Build history of the part. All positions in model axes, mm. Face numbers are marked on the shaded views. A direction names the side the tool comes from. Round coordinates to 2 decimals unless told otherwise and drop trailing zeros. Write each loop counter-clockwise with the first axis right and the second up, starting at its lowest first coordinate (ties: lowest second). Pieces come first, ordered by that corner, then holes. Notation, with made-up numbers: (85, 15.5) -> (125, 15.5) arc R7 ccw to (125, 28.5) -> close; hole circle Ø7 at (53.25, 53.25). An arc over 180 degrees is marked (long way). Return JSON: item names as keys, results as strings.
from build123d import *

# Parameters (mm, degrees)
F2_R     = 46.0375
F3_DEPTH = 19.05
F3_TAPER = 15
F0_R     = 41.275
F4_DEPTH = 25.4
F5_R     = 46.0375
F6_DEPTH = 1.5875


with BuildPart() as f3:
    # F2 (on offset) → F3 (new body)
    with BuildSketch(Plane.XY.offset(-41.275)):
        Circle(F2_R)
    extrude(amount=F3_DEPTH, taper=F3_TAPER)

    # F0 (on Top) → F4 (join)
    with BuildSketch(Plane.XY):
        Circle(F0_R)
    extrude(amount=-F4_DEPTH)

    # F5 (on face) → F6 (join)
    with BuildSketch(Plane(origin=(0, 0, -41.275), x_dir=(1, 0, 0), z_dir=(0, 0, -1))):
        Polygon((101.6, -101.6), (101.6, 0), (101.6, 101.6), (-101.6, 101.6), (-101.6, -101.6), align=None)
        Circle(F5_R, mode=Mode.SUBTRACT)
        Circle(F5_R)
    extrude(amount=F6_DEPTH)


solid = f3.part
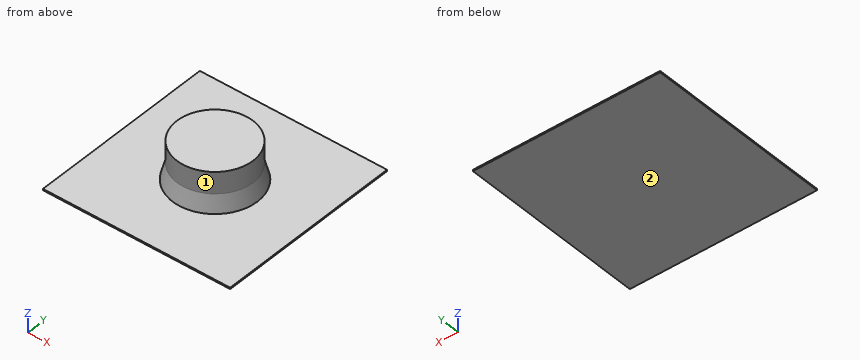
Q1. Saw through at D-D on y = 71. List the corners of the cut face in (x, z) (1 decimal).
Verdict:
{"outline": "(-101.6, -42.9) -> (101.6, -42.9) -> (101.6, -41.3) -> (-101.6, -41.3) -> close"}
Q2. Saw through at C-C on z = -5. List the corners of the cut face in (x, y) (3 decimals), then the cut area to 3 significant figures.
Verdict:
{"outline": "circle Ø82.55 at (0, 0)", "area": "5,350 mm²"}
Q3. Pin check, flat tips, straight feed: pin 1 Ø3 at (x, z) = (14.5, -23) entering from -Y; pin 2 Ø4 at (x, z) = (-20.5, -15) entering from -Y. Stop position of each tip, or through.
Verdict:
{"pin 1": "stops at y = -39.19", "pin 2": "stops at y = -36.9"}
Q4. 3-axis set-ups, long thin cutter, end or side, ignore diameter. For the marked faces 1 and 2: which of +Z, -Z, +X, -X, +Y, -Y reach the whole face in a straight line?
Verdict:
{"face 1": "+Z", "face 2": "-Z, +X, -X, +Y, -Y"}
Q5. Saw through at A-A on y = 0. List the corners of the cut face in (x, z) (1 decimal), then the cut area to 3 significant figures.
Verdict:
{"outline": "(-101.6, -42.9) -> (101.6, -42.9) -> (101.6, -41.3) -> (46, -41.3) -> (41.3, -23.5) -> (41.3, 0) -> (-41.3, 0) -> (-41.3, -23.5) -> (-46, -41.3) -> (-101.6, -41.3) -> close", "area": "3,810 mm²"}
Q6. Wall check: L1, parallel to Z at x = -33, y = 47 (1 decimal); L2, parallel to Y at x = -30.5, z = -25; L3, parallel to Y at x = -14.5, z = -3. Give the ranges that are in metal, low to high.
Verdict:
{"L1": "z = -42.9 to -41.3", "L2": "y = -28.4 to 28.4", "L3": "y = -38.64 to 38.64"}
